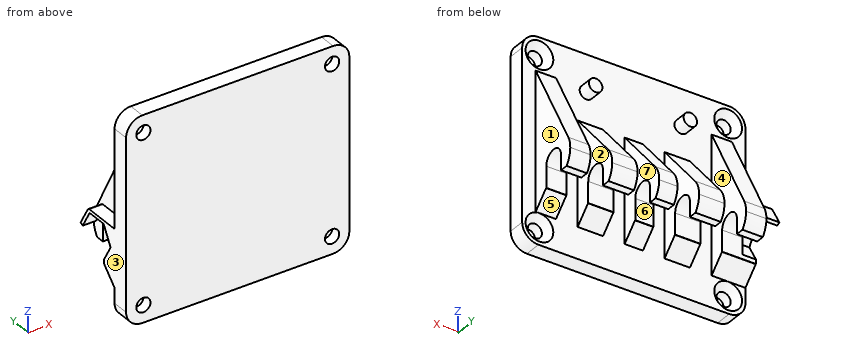
```python
from build123d import *

# Parameters (mm, degrees)
SKETCH4_W           = 6.4
SKETCH4_H           = 40
SKETCH4_W_2         = 5.4
SKETCH4_W_3         = 7.5
BOSS_EXTRUDE4_DEPTH = 5
SKETCH6_W           = 5.4
SKETCH6_H           = 40
SKETCH6_W_2         = 7.5
BOSS_EXTRUDE5_DEPTH = 15
SKETCH7_R           = 3.2
CUT_EXTRUDE2_DEPTH  = 73.625684162
CUT_EXTRUDE3_REACH  = 74.626
CUT_EXTRUDE4_REACH  = 90.566
CUT_EXTRUDE5_REACH  = 92.449
SKETCH10_R          = 2.1
CHAMFER1_SIZE       = 2
FILLET1_R           = 4.8
SKETCH11_R          = 2
BOSS_EXTRUDE6_DEPTH = 4
BOSS_EXTRUDE7_DEPTH = 4
CUT_EXTRUDE6_DEPTH  = 89.566359302
CHAMFER2_SIZE       = 4.5


with BuildPart() as part:
    # Sketch4 → Boss-Extrude4 (new body)
    with BuildSketch(Plane(origin=(0, 0, 0), x_dir=(1, 0, 0), z_dir=(0, 1, 0))):
        Polygon((0, 60), (0, 0), (66, 0), (66, 60), (56, 60), (56, 50), (62, 50), (62, 10), (56, 10), (56, 20), (49.6, 20), (42.1, 20), (35.7, 20), (30.3, 20), (30.3, 60), align=None)
        with Locations((38.9, 40)):
            Rectangle(SKETCH4_W, SKETCH4_H)
        with Locations((33, 40)):
            Rectangle(SKETCH4_W_2, SKETCH4_H)
        with Locations((45.85, 40)):
            Rectangle(SKETCH4_W_3, SKETCH4_H)
        Polygon((56, 50), (56, 60), (49.6, 60), (49.6, 20), (56, 20), align=None)
        Polygon((62, 50), (56, 50), (56, 20), (56, 10), (62, 10), align=None)
    extrude(amount=BOSS_EXTRUDE4_DEPTH)

    # Sketch6 → Boss-Extrude5 (add)
    with BuildSketch(Plane(origin=(0, 5, 0), x_dir=(1, 0, 0), z_dir=(0, 1, 0))):
        with Locations((33, 40)):
            Rectangle(SKETCH6_W, SKETCH6_H)
        with Locations((45.85, 40)):
            Rectangle(SKETCH6_W_2, SKETCH6_H)
        Polygon((62, 50), (56, 50), (56, 20), (56, 10), (62, 10), align=None)
    boss_extrude5 = extrude(amount=BOSS_EXTRUDE5_DEPTH)

    # Sketch7 → Cut-Extrude2 (cut, through all)
    with BuildSketch(Plane.ZY.offset(-30.3)):
        with Locations(Location((-40, 12.8, 0), (0, 0, 180))):
            Circle(SKETCH7_R)
    cut_extrude2 = extrude(amount=-CUT_EXTRUDE2_DEPTH, mode=Mode.SUBTRACT)

    # Cut-Extrude3: up to this face of the body (flat: up to its plane)
    cut_extrude3_end = Plane(part.part.faces().sort_by_distance((49.6, 12.5, -20.427200187))[0])
    # Sketch8 → Cut-Extrude3 (cut, up to the picked face)
    with BuildSketch(Plane.ZY.offset(-30.3), mode=Mode.PRIVATE) as cut_extrude3_sk1:
        with BuildLine():
            Line((-60, 20), (-60, 5))
            Line((-60, 5), (-44.714360106, 18.241948989))
            ThreePointArc((-44.714360106, 18.241948989), (-42.515747134, 19.546185319), (-40, 20))
            Line((-40, 20), (-60, 20))
        make_face()
    cut_extrude3_tool1 = split(extrude(cut_extrude3_sk1.sketch, amount=-CUT_EXTRUDE3_REACH, mode=Mode.PRIVATE), bisect_by=cut_extrude3_end, keep=Keep.BOTH, mode=Mode.PRIVATE)
    # Sketch8 → Cut-Extrude3 (cut, up to the picked face)
    with BuildSketch(Plane.ZY.offset(-30.3), mode=Mode.PRIVATE) as cut_extrude3_sk2:
        with BuildLine():
            Line((-35.285639894, 18.241948989), (-20, 5))
            Line((-20, 5), (-20, 20))
            Line((-20, 20), (-40, 20))
            ThreePointArc((-40, 20), (-37.484252866, 19.546185319), (-35.285639894, 18.241948989))
        make_face()
    cut_extrude3_tool2 = split(extrude(cut_extrude3_sk2.sketch, amount=-CUT_EXTRUDE3_REACH, mode=Mode.PRIVATE), bisect_by=cut_extrude3_end, keep=Keep.BOTH, mode=Mode.PRIVATE)
    cut_extrude3_1 = cut_extrude3_tool1.solids().sort_by(Axis((30.3, 15.029403, -54.154339), (1, 0, 0)))[0]
    add(cut_extrude3_1, mode=Mode.SUBTRACT)
    cut_extrude3_2 = cut_extrude3_tool2.solids().sort_by(Axis((30.3, 15.029403, -25.845661), (1, 0, 0)))[0]
    add(cut_extrude3_2, mode=Mode.SUBTRACT)
    cut_extrude3 = cut_extrude3_1 + cut_extrude3_2  # Cut-Extrude3 as one shape, for the pattern or mirror that repeats it

    # Sketch9 → Cut-Extrude4 (cut, up to next)
    with BuildSketch(Plane(origin=(62, 0, 0), x_dir=(0, 0, -1), z_dir=(1, 0, 0)), mode=Mode.PRIVATE) as cut_extrude4_sk1:
        with BuildLine():
            ThreePointArc((36.619205024, 19.156903753), (38.257832819, 19.786047059), (40, 20))
            Line((40, 20), (10, 20))
            Line((10, 20), (10, 5))
            Line((10, 5), (36.619205024, 19.156903753))
        make_face()
    cut_extrude4_tool1 = extrude(cut_extrude4_sk1.sketch, amount=-CUT_EXTRUDE4_REACH, mode=Mode.PRIVATE) & part.part
    # Sketch9 → Cut-Extrude4 (cut, up to next)
    with BuildSketch(Plane(origin=(62, 0, 0), x_dir=(0, 0, -1), z_dir=(1, 0, 0)), mode=Mode.PRIVATE) as cut_extrude4_sk2:
        with BuildLine():
            ThreePointArc((40, 20), (44.259746459, 18.604701552), (46.868488023, 14.959600029))
            Line((46.868488023, 14.959600029), (50, 5))
            Line((50, 5), (50, 20))
            Line((50, 20), (40, 20))
        make_face()
    cut_extrude4_tool2 = extrude(cut_extrude4_sk2.sketch, amount=-CUT_EXTRUDE4_REACH, mode=Mode.PRIVATE) & part.part
    cut_extrude4_1 = cut_extrude4_tool1.solids().sort_by_distance((62, 15.005893, -19.424487))[0]
    add(cut_extrude4_1, mode=Mode.SUBTRACT)
    cut_extrude4_2 = cut_extrude4_tool2.solids().sort_by_distance((62, 15.504148, -47.92116))[0]
    add(cut_extrude4_2, mode=Mode.SUBTRACT)
    cut_extrude4 = cut_extrude4_1 + cut_extrude4_2  # Cut-Extrude4 as one shape, for the pattern or mirror that repeats it

    # Mirror1: Boss-Extrude5, Cut-Extrude2, Cut-Extrude3, Cut-Extrude4 across plane
    add(boss_extrude5.mirror(Plane.ZY.offset(-33)))
    add(cut_extrude2.mirror(Plane.ZY.offset(-33)), mode=Mode.SUBTRACT)
    add(cut_extrude3.mirror(Plane.ZY.offset(-33)), mode=Mode.SUBTRACT)
    add(cut_extrude4.mirror(Plane.ZY.offset(-33)), mode=Mode.SUBTRACT)

    # Sketch10 → Cut-Extrude5 (cut, up to next)
    with BuildSketch(Plane(origin=(0, 5, 0), x_dir=(1, 0, 0), z_dir=(0, 1, 0)), mode=Mode.PRIVATE) as cut_extrude5_sk1:
        with Locations(Location((5.1, 54.9, 0), (0, 0, 270))):
            Circle(SKETCH10_R)
    cut_extrude5_tool1 = extrude(cut_extrude5_sk1.sketch, amount=-CUT_EXTRUDE5_REACH, mode=Mode.PRIVATE) & part.part
    # Sketch10 → Cut-Extrude5 (cut, up to next)
    with BuildSketch(Plane(origin=(0, 5, 0), x_dir=(1, 0, 0), z_dir=(0, 1, 0)), mode=Mode.PRIVATE) as cut_extrude5_sk2:
        with Locations(Location((60.9, 54.9, 0), (0, 0, 270))):
            Circle(SKETCH10_R)
    cut_extrude5_tool2 = extrude(cut_extrude5_sk2.sketch, amount=-CUT_EXTRUDE5_REACH, mode=Mode.PRIVATE) & part.part
    # Sketch10 → Cut-Extrude5 (cut, up to next)
    with BuildSketch(Plane(origin=(0, 5, 0), x_dir=(1, 0, 0), z_dir=(0, 1, 0)), mode=Mode.PRIVATE) as cut_extrude5_sk3:
        with Locations(Location((60.9, 5.1, 0), (0, 0, 270))):
            Circle(SKETCH10_R)
    cut_extrude5_tool3 = extrude(cut_extrude5_sk3.sketch, amount=-CUT_EXTRUDE5_REACH, mode=Mode.PRIVATE) & part.part
    # Sketch10 → Cut-Extrude5 (cut, up to next)
    with BuildSketch(Plane(origin=(0, 5, 0), x_dir=(1, 0, 0), z_dir=(0, 1, 0)), mode=Mode.PRIVATE) as cut_extrude5_sk4:
        with Locations(Location((5.1, 5.1, 0), (0, 0, 270))):
            Circle(SKETCH10_R)
    cut_extrude5_tool4 = extrude(cut_extrude5_sk4.sketch, amount=-CUT_EXTRUDE5_REACH, mode=Mode.PRIVATE) & part.part
    add(cut_extrude5_tool1.solids().sort_by_distance((5.1, 5, -54.9))[0], mode=Mode.SUBTRACT)
    add(cut_extrude5_tool2.solids().sort_by_distance((60.9, 5, -54.9))[0], mode=Mode.SUBTRACT)
    add(cut_extrude5_tool3.solids().sort_by_distance((60.9, 5, -5.1))[0], mode=Mode.SUBTRACT)
    add(cut_extrude5_tool4.solids().sort_by_distance((5.1, 5, -5.1))[0], mode=Mode.SUBTRACT)

    # Chamfer1
    chamfer1_edges = [part.edges().sort_by_distance(p)[0] for p in [
        (5.1, 5, -7.2),
        (60.9, 5, -7.2),
        (60.9, 5, -57),
        (5.1, 5, -57),
    ]]
    chamfer(chamfer1_edges, length=CHAMFER1_SIZE)

    # Fillet1
    fillet1_edges = [part.edges().sort_by_distance(p)[0] for p in [
        (66, 2.5, 0),
        (0, 2.5, 0),
        (0, 2.5, -60),
        (66, 2.5, -60),
    ]]
    fillet(fillet1_edges, radius=FILLET1_R)

    # Sketch11 → Boss-Extrude6 (add)
    with BuildSketch(Plane(origin=(0, 5, 0), x_dir=(1, 0, 0), z_dir=(0, 1, 0))):
        with Locations(Location((19, 11, 0), (0, 0, 270))):
            Circle(SKETCH11_R)
        with Locations(Location((47, 11, 0), (0, 0, 270))):
            Circle(SKETCH11_R)
    extrude(amount=BOSS_EXTRUDE6_DEPTH)

    # Sketch12 → Boss-Extrude7 (add)
    with BuildSketch(Plane.ZY.offset(-4)):
        with BuildLine():
            Line((-39.5, 19.72820323), (-40, 18.862177826))
            Line((-40, 18.862177826), (-34.75, 15.831088913))
            Line((-34.75, 15.831088913), (-34.75, 9.768911087))
            Line((-34.75, 9.768911087), (-40, 6.737822174))
            Line((-40, 6.737822174), (-44.957437416, 9.6))
            Line((-44.957437416, 9.6), (-46.25, 9.6))
            Line((-46.25, 9.6), (-46.25, 5))
            Line((-46.25, 5), (-33.75, 5))
            Line((-33.75, 5), (-33.75, 15.831088913))
            ThreePointArc((-33.75, 15.831088913), (-33.883974596, 16.331088913), (-34.25, 16.697114317))
            Line((-34.25, 16.697114317), (-39.5, 19.72820323))
        make_face()
    extrude(amount=BOSS_EXTRUDE7_DEPTH)

    # Sketch15 → Cut-Extrude6 (cut, through all)
    with BuildSketch(Plane.ZY.offset(-4)):
        with BuildLine():
            ThreePointArc((-40, 9.6), (-43.2, 12.8), (-40, 16))
            Line((-40, 16), (-44.5, 16))
            Line((-44.5, 16), (-46.449806199, 16))
            ThreePointArc((-46.449806199, 16), (-46.679434726, 15.487964236), (-46.868488023, 14.959600029))
            Line((-46.868488023, 14.959600029), (-48.553661286, 9.6))
            Line((-48.553661286, 9.6), (-46.25, 9.6))
            Line((-46.25, 9.6), (-44.957437416, 9.6))
            Line((-44.957437416, 9.6), (-40, 9.6))
        make_face()
        with BuildLine():
            ThreePointArc((-46.868488023, 14.959600029), (-46.679434726, 15.487964236), (-46.449806199, 16))
            Line((-46.449806199, 16), (-47.302319396, 16))
            Line((-47.302319396, 16), (-54.690060838, 9.6))
            Line((-54.690060838, 9.6), (-48.553661286, 9.6))
            Line((-48.553661286, 9.6), (-46.868488023, 14.959600029))
        make_face()
        Polygon((-48.553661286, 9.6), (-54.690060838, 9.6), (-60, 5), (-55.2, 5), (-50, 5), align=None)
        Polygon((-46.25, 5), (-46.25, 9.6), (-48.553661286, 9.6), (-50, 5), align=None)
        with BuildLine():
            Line((-46.449806199, 16), (-44.5, 16))
            Line((-44.5, 16), (-44.5, 18.420498199))
            ThreePointArc((-44.5, 18.420498199), (-44.608044921, 18.332261925), (-44.714360106, 18.241948989))
            ThreePointArc((-44.714360106, 18.241948989), (-45.693525809, 17.207239937), (-46.449806199, 16))
        make_face()
        with BuildLine():
            Line((-47.302319396, 16), (-46.449806199, 16))
            ThreePointArc((-46.449806199, 16), (-45.693525809, 17.207239937), (-44.714360106, 18.241948989))
            Line((-44.714360106, 18.241948989), (-47.302319396, 16))
        make_face()
    extrude(amount=-CUT_EXTRUDE6_DEPTH, mode=Mode.SUBTRACT)

    # Chamfer2
    chamfer2_edges = [part.edges().sort_by_distance(p)[0] for p in [
        (5, 5, -46.25),
        (33, 5, -46.25),
        (45.85, 5, -46.25),
        (20.15, 5, -46.25),
        (59, 5, -46.25),
    ]]
    chamfer(chamfer2_edges, length=CHAMFER2_SIZE)


solid = part.part
```
Could you check a few things on this model? Use its own coordinates, in mm. Face numbers are marked on the shaded views. A direction names the side the tool comes from. Coordinates: 2 decimals unless noted, no trailing zeros. Order: outer loops, then holes, each group sorted by start corner. A loop starts at its lowest first (then second) coordinate and runs counter-clockwise, first axis right, second up. Notation, with made-up numbers: M 38.25,-26.75 L 52.25,-26.75 A17 ccw 52.25,-9.75 Z; hole C -37,-21.75 d11. An arc over 180 degrees is marked long. Use a Markdown table: item, result. Add a question column.
Q1. Which directions (+Z, -Z, +X, -X, +Y, -Y) give clear straight access to the entire face, cutting with the end or side of a thin tool? Please do the marked faces 5, 6 and 7.
Q2. I want a section at C-C on z = -29. List the corners of the cut face in (x, y) for me.
Q3. We'd pull the mould along X, two halves only. Please class the marked faces 1, 2, 3 and 4: pulls with the +X half, pulls with the -X half, needs draft (parallel to the pull), parting line crosses it, or undercut.
Q4. I'm going to push flat-ended pins straight in: pin 1 (1.9 mm diameter, centred on x = 21, z = -43.5, fed in from +Y); pin 2 (2.5 mm diameter, centred on x = 8, y = 17.5, fed in from -Z); pin 3 (2 mm diameter, centred on x = 9.5, y = 11, fed in from +Z). Where does each tip first touch, or does it pass through?
Q5. I want a section at B-B on x = 44. List the corners of the cut face in (y, z) for me, then the cut area to 3 significant figures.
Q6. I want a section at A-A on y = 17.5. List the corners of the cut face in (x, z) for me.
Q7. If I drill on L1, parallel to X at y = 2, z = -5.1; L2, parallel to Z at x = 46.5, y = 5.25; L3, parallel to Y at x = 16.5, z = -3.5, over which ranges is the centre line in solid material (lowest first)?
Q8. I want a section at D-D on z = -41. Give the number of separate pieces and of enclosed holes in the cut face, then the cut area to 3 significant figures.
Checked values:
| question | item | result |
|---|---|---|
| 1 | face 5 | -Z, +X, -X, +Y |
| 1 | face 6 | -Z, +X, -X |
| 1 | face 7 | +Z, -Z, +Y |
| 2 | outline | M 0,0 L 66,0 L 66,5 L 62,5 L 62,15.1 L 56,15.1 L 56,5 L 49.6,5 L 49.6,12.8 L 42.1,12.8 L 42.1,5 L 35.7,5 L 35.7,12.8 L 30.3,12.8 L 30.3,5 L 23.9,5 L 23.9,12.8 L 16.4,12.8 L 16.4,5 L 10,5 L 10,15.1 L 4,15.1 L 4,5 L 0,5 Z |
| 3 | face 1 | pulls with the +X half |
| 3 | face 2 | undercut |
| 3 | face 3 | pulls with the -X half |
| 3 | face 4 | undercut |
| 4 | pin 1 | y = 19.53 |
| 4 | pin 2 | z = -44.5 |
| 4 | pin 3 | z = -19.4 |
| 5 | outline | M 0,-60 L 5,-60 L 5,-50.75 L 9.5,-46.25 L 9.6,-46.25 L 9.6,-40 A3.2 cw 16,-40 L 16,-44.5 L 18.42,-44.5 A7.2 ccw 18.24,-35.29 L 5,-20 L 5,0 L 0,0 Z |
| 5 | area | 508 mm² |
| 6 | outline | M 0,-37.64 L 4,-37.64 L 4,-44.5 L 10,-44.5 L 10,-33.5 L 4,-33.5 L 4,-35.64 L 0,-35.64 Z; M 16.4,-44.5 L 23.9,-44.5 L 23.9,-34.43 L 16.4,-34.43 Z; M 30.3,-44.5 L 35.7,-44.5 L 35.7,-34.43 L 30.3,-34.43 Z; M 42.1,-44.5 L 49.6,-44.5 L 49.6,-34.43 L 42.1,-34.43 Z; M 56,-44.5 L 62,-44.5 L 62,-33.5 L 56,-33.5 Z |
| 7 | L1 | 0 to 3, 7.2 to 58.8, 63 to 66 |
| 7 | L2 | -50.5 to -20.29, -12.94 to -9.06 |
| 7 | L3 | 0 to 5 |
| 8 | separate pieces | 6 |
| 8 | enclosed holes | 0 |
| 8 | area | 616 mm² |
